CAD build for the part. Positions are in the model's coordinates, mm. Face numbers are marked on the shaded views. A direction names the side the tool comes from. Coordinates: 2 decimals unless noted, no trailing zeros. Order: outer loops, then holes, each group sorted by start corner. A loop starts at its lowest first (then second) coordinate and runs counter-clockwise, first axis right, second up. Notation, with made-up numbers: M 53,-5.5 L 75,-5.5 A27 ccw 75,10.5 Z; hole C 68,9 d6. An arc over 180 degrees is marked long. Write item = value, one per line.
from build123d import *

# Parameters (mm, degrees)
F2_R     = 6
F3_DEPTH = 40.001
F4_R     = 6
F5_DEPTH = 40.001
F6_DEPTH = 40.001


with BuildPart() as f1:
    # F0 (on Front) → F1 (revolve)
    with BuildSketch(Plane.XZ):
        Polygon((-406.362363, 30), (-406.362363, 0), (-312.251694, 0), (-296.473032, 0), (-266.237753, 0), (-266.237753, 15), (-276.237753, 25), (-376.362363, 25), (-376.362363, 40), (-396.362363, 40), align=None)
    revolve(axis=Axis((-281.355392, 0, 0), (-1, 0, 0)))

    # F2 (on Front) → F3 (cut, through all)
    with BuildSketch(Plane.XZ):
        with Locations((-304.362363, 0)):
            Circle(F2_R)
    extrude(amount=-F3_DEPTH, mode=Mode.SUBTRACT)

    # F4 (on face) → F5 (cut, through all)
    with BuildSketch(Plane(origin=(0, 0, 0), x_dir=(-1, 0, 0), z_dir=(0, 1, 0))):
        with Locations((304.362363, 0)):
            Circle(F4_R)
    extrude(amount=-F5_DEPTH, mode=Mode.SUBTRACT)

    # F2 (on Front) → F6 (cut, through all)
    with BuildSketch(Plane.XZ):
        with Locations((-304.362363, 0)):
            Circle(F2_R)
    extrude(amount=F6_DEPTH, mode=Mode.SUBTRACT)


solid = f1.part
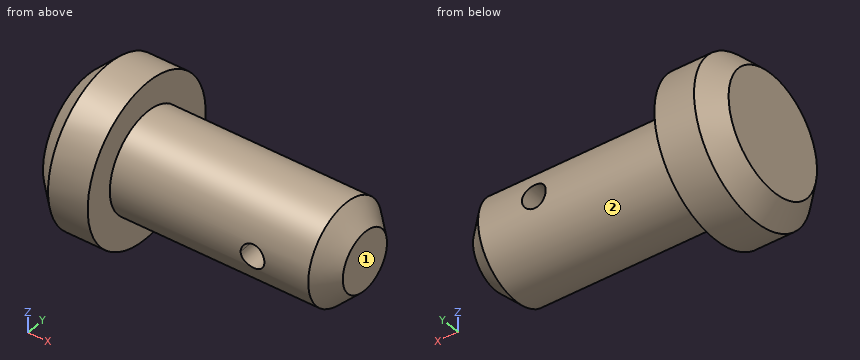
(1) Pin check, flat tips, straight feed: pin 1 Ø1 at (x, y) = (-388.5, 31) entering from -Z; pin 2 Ø1 at (x, y) = (-282, -19) entering from -Z; pin 3 Ø4 at (x, z) = (-371, 2.5) entering from -Y (3 decimals); pin 4 Ø7 at (x, z) = (-304.36, 0) entering from +Y. Stop position of each tip, or through.
Evaluation:
pin_1 = -25.88
pin_2 = -16.82
pin_3 = -24.995
pin_4 = through
(2) Slice it at A-A, the plane x = -286.5. Write the cut outline in (y, z).
Evaluation:
outline = C 0,0 d50
(3) Wall check: line 1 (X direction, y = 15, z = 0); line 2 (Z direction, x = -351.5, y = -0.5) (3 decimals); line 3 (X direction, y = 19.25, z = 0). Give the ranges that are in metal, low to high. Write a range as from..to.
Evaluation:
line_1 = -406.36..-310.36, -298.36..-266.24
line_2 = -24.995..24.995
line_3 = -406.36..-310.36, -298.36..-270.49
(4) Tool access for the marked faces 1 and 2: list every direction of +Z, -Z, +X, -X, +Y, -Y with a clear straight run to the whole face (end or side of a thin tool).
Evaluation:
face_1 = +Z, -Z, +X, +Y, -Y
face_2 = +X
